Verification items for the finished model (mm, model axes). Face numbers are marked on the shaded views. A direction names the side the tool comes from. Give positions to 0.01 mm unless a question says otherwise; leave off trailing zeros. Order: outer loops, then holes, each group sorted by start corner. A loop starts at its lowest first (then second) coordinate and runs counter-clockwise, first axis right, second up.
(1) Sectioned sample at B-B on z = -0.75. Record the cut outline in (x, y).
(2) Access from +Z, -Z, +X, -X, +Y, -Y to the whole of each face (thin tool, end or side, straight path). Record for the marked faces 5, 6 and 7.
(3) Gauge pin test, flat ends, axial feed: pin 1 (3.5 mm diameter, centred on x = 5, y = -11.5, fed in from -Z); pin 2 (1.3 mm diameter, centred on y = 12, z = -3, fed in from -X); pin 3 (3.5 mm diameter, centred on y = 1.5, z = -0.5, fed in from -X); pin 4 (2 mm diameter, centred on x = 2, z = -3.5, fed in from -Y). Record the tip position at first contact, or that the pin passes through.
(4) Sectioned sample at A-A on x = -9.75. Record the cut outline in (y, z).
(5) Sectioned sample at D-D on x = 7. Record the cut outline in (y, z), plus the area to 3 significant figures.
(6) Mould release check, pull along Y, two halves, no side actions. Record for the marked faces 1, 2, 3 and 4: pulls with the +Y half, pulls with the -Y half, needs draft (parallel to the pull), parting line crosses it, or undercut.
(7) Sectioned sample at C-C on x = 3. Record the cut outline in (y, z), plus the area to 3 significant figures.
(8) Scan lines: L1, parallel to Y at x = 12.5, z = 0; L2, parallel to Y at x = -9.75, z = -4.25; L3, parallel to X at y = -1.25, z = 1.25. Record each from-to range of solid material in increasing order.
```python
from build123d import *

# Parameters (mm, degrees)
SKETCH1_W           = 30
SKETCH1_H           = 22
BOSS_EXTRUDE1_DEPTH = 2
SKETCH2_W           = 13
SKETCH2_H           = 20
CUT_EXTRUDE1_DEPTH  = 2
FILLET1_R           = 3
SKETCH3_W           = 30
SKETCH3_H           = 22
BOSS_EXTRUDE2_DEPTH = 20
SKETCH4_W           = 30
SKETCH4_H           = 22
BOSS_EXTRUDE3_DEPTH = 2
SKETCH5_W           = 30
SKETCH5_H           = 22
BOSS_EXTRUDE4_DEPTH = 2
SKETCH6_W           = 18.015144258
SKETCH6_H           = 26
CUT_EXTRUDE2_DEPTH  = 1.2
SKETCH7_W           = 18
SKETCH7_H           = 26
CUT_EXTRUDE3_DEPTH  = 1.2
SKETCH8_W           = 27.6
SKETCH8_H           = 18
CUT_EXTRUDE4_DEPTH  = 1.2
SKETCH9_W           = 27.6
SKETCH9_H           = 18.015144258
CUT_EXTRUDE5_DEPTH  = 1.2
SKETCH10_W          = 8.9
SKETCH10_H          = 1
CUT_EXTRUDE7_DEPTH  = 1.8
SKETCH12_W          = 5.2
SKETCH12_H          = 1.2
CUT_EXTRUDE8_DEPTH  = 1.8
CUT_EXTRUDE9_DEPTH  = 3.2
SKETCH14_W          = 2.8
SKETCH14_H          = 1
CUT_EXTRUDE10_DEPTH = 5
SKETCH15_W          = 8.9
SKETCH15_H          = 1
CUT_EXTRUDE11_DEPTH = 5
SKETCH16_W          = 5.1
SKETCH16_H          = 1.2
CUT_EXTRUDE12_DEPTH = 5
SKETCH17_W          = 27.6
SKETCH17_H          = 14.5
CUT_EXTRUDE13_DEPTH = 23.6
CUT_EXTRUDE14_DEPTH = 5
SKETCH19_W          = 2.8
SKETCH19_H          = 20
CUT_EXTRUDE16_DEPTH = 3.5
SKETCH20_W          = 8.574892863
SKETCH20_H          = 20
SKETCH20_W_2        = 12.614156469
CUT_EXTRUDE18_DEPTH = 5
SKETCH24_W          = 0.5
SKETCH24_H          = 26
CUT_EXTRUDE19_DEPTH = 100
SKETCH25_W          = 4.142834468
SKETCH25_H          = 28.533772401
SKETCH25_W_2        = 4.453547053
SKETCH25_H_2        = 29.155197571
CUT_EXTRUDE20_DEPTH = 3.5


with BuildPart() as part:
    # Sketch1 → Boss-Extrude1 (new body)
    with BuildSketch(Plane.XY):
        with Locations((1.554069904, 0.785714286)):
            Rectangle(SKETCH1_W, SKETCH1_H)
    extrude(amount=BOSS_EXTRUDE1_DEPTH)

    # Sketch2 → Cut-Extrude1 (cut)
    with BuildSketch(Plane.XY.offset(2)):
        with Locations((-5.945930096, 0.785714286)):
            Rectangle(SKETCH2_W, SKETCH2_H)
        with Locations((9.054069904, 0.785714286)):
            Rectangle(SKETCH2_W, SKETCH2_H)
    extrude(amount=-CUT_EXTRUDE1_DEPTH, mode=Mode.SUBTRACT)

    # Fillet1
    fillet1_edges = [part.edges().sort_by_distance(p)[0] for p in [
        (-12.445930096, -9.214285714, 1),
        (-12.445930096, 10.785714286, 1),
        (0.554069904, 10.785714286, 1),
        (0.554069904, -9.214285714, 1),
        (15.554069904, 10.785714286, 1),
        (15.554069904, -9.214285714, 1),
        (2.554069904, -9.214285714, 1),
        (2.554069904, 10.785714286, 1),
    ]]
    fillet(fillet1_edges, radius=FILLET1_R)

    # Sketch3 → Boss-Extrude2 (add)
    with BuildSketch(Plane(origin=(0, 0, 0), x_dir=(-1, 0, 0), z_dir=(0, 0, -1))):
        with Locations((-1.554069904, 0.785714286)):
            Rectangle(SKETCH3_W, SKETCH3_H)
    extrude(amount=BOSS_EXTRUDE2_DEPTH)

    # Sketch4 → Boss-Extrude3 (add)
    with BuildSketch(Plane(origin=(0, 11.785714286, 0), x_dir=(1, 0, 0), z_dir=(0, 1, 0))):
        with Locations((1.554069904, 9)):
            Rectangle(SKETCH4_W, SKETCH4_H)
    extrude(amount=BOSS_EXTRUDE3_DEPTH)

    # Sketch5 → Boss-Extrude4 (add)
    with BuildSketch(Plane(origin=(0, -10.214285714, 0), x_dir=(-1, 0, 0), z_dir=(0, -1, 0))):
        with Locations((-1.554069904, 9)):
            Rectangle(SKETCH5_W, SKETCH5_H)
    extrude(amount=BOSS_EXTRUDE4_DEPTH)

    # Sketch6 → Cut-Extrude2 (cut)
    with BuildSketch(Plane(origin=(16.554069904, 0, 0), x_dir=(0, 0, -1), z_dir=(1, 0, 0))):
        with Locations((10.992427871, 0.785714286)):
            Rectangle(SKETCH6_W, SKETCH6_H)
    extrude(amount=-CUT_EXTRUDE2_DEPTH, mode=Mode.SUBTRACT)

    # Sketch7 → Cut-Extrude3 (cut)
    with BuildSketch(Plane.ZY.offset(13.445930096)):
        with Locations((-11, 0.785714286)):
            Rectangle(SKETCH7_W, SKETCH7_H)
    extrude(amount=-CUT_EXTRUDE3_DEPTH, mode=Mode.SUBTRACT)

    # Sketch8 → Cut-Extrude4 (cut)
    with BuildSketch(Plane(origin=(0, 13.785714286, 0), x_dir=(1, 0, 0), z_dir=(0, 1, 0))):
        with Locations((1.554069904, 11)):
            Rectangle(SKETCH8_W, SKETCH8_H)
    extrude(amount=-CUT_EXTRUDE4_DEPTH, mode=Mode.SUBTRACT)

    # Sketch9 → Cut-Extrude5 (cut)
    with BuildSketch(Plane.XZ.offset(12.214285714)):
        with Locations((1.554069904, -10.992427871)):
            Rectangle(SKETCH9_W, SKETCH9_H)
    extrude(amount=-CUT_EXTRUDE5_DEPTH, mode=Mode.SUBTRACT)

    # Sketch10 → Cut-Extrude7 (cut)
    with BuildSketch(Plane(origin=(0, 12.585714286, 0), x_dir=(1, 0, 0), z_dir=(0, 1, 0))):
        with Locations((-7.795930096, 2.5)):
            Rectangle(SKETCH10_W, SKETCH10_H)
        with Locations((10.904069904, 2.5)):
            Rectangle(SKETCH10_W, SKETCH10_H)
    extrude(amount=-CUT_EXTRUDE7_DEPTH, mode=Mode.SUBTRACT)

    # Sketch12 → Cut-Extrude8 (cut)
    with BuildSketch(Plane(origin=(0, 12.585714286, 0), x_dir=(1, 0, 0), z_dir=(0, 1, 0))):
        with Locations((-5.945930096, 2.6)):
            Rectangle(SKETCH12_W, SKETCH12_H)
        with Locations((9.054069904, 2.6)):
            Rectangle(SKETCH12_W, SKETCH12_H)
    extrude(amount=-CUT_EXTRUDE8_DEPTH, mode=Mode.SUBTRACT)

    # Sketch13 → Cut-Extrude9 (cut)
    with BuildSketch(Plane.XY):
        with BuildLine():
            Line((-9.445930096, 10.785714286), (-2.445930096, 10.785714286))
            ThreePointArc((-2.445930096, 10.785714286), (-0.324609753, 9.907034629), (0.554069904, 7.785714286))
            Line((0.554069904, 7.785714286), (0.554069904, -6.214285714))
            ThreePointArc((0.554069904, -6.214285714), (-0.324609753, -8.335606058), (-2.445930096, -9.214285714))
            Line((-2.445930096, -9.214285714), (-9.445930096, -9.214285714))
            ThreePointArc((-9.445930096, -9.214285714), (-11.56725044, -8.335606058), (-12.445930096, -6.214285714))
            Line((-12.445930096, -6.214285714), (-12.445930096, 7.785714286))
            ThreePointArc((-12.445930096, 7.785714286), (-11.56725044, 9.907034629), (-9.445930096, 10.785714286))
        make_face()
        with BuildLine():
            Line((5.554069904, 10.785714286), (12.554069904, 10.785714286))
            ThreePointArc((12.554069904, 10.785714286), (14.675390247, 9.907034629), (15.554069904, 7.785714286))
            Line((15.554069904, 7.785714286), (15.554069904, -6.214285714))
            ThreePointArc((15.554069904, -6.214285714), (14.675390247, -8.335606058), (12.554069904, -9.214285714))
            Line((12.554069904, -9.214285714), (5.554069904, -9.214285714))
            ThreePointArc((5.554069904, -9.214285714), (3.43274956, -8.335606058), (2.554069904, -6.214285714))
            Line((2.554069904, -6.214285714), (2.554069904, 7.785714286))
            ThreePointArc((2.554069904, 7.785714286), (3.43274956, 9.907034629), (5.554069904, 10.785714286))
        make_face()
    extrude(amount=-CUT_EXTRUDE9_DEPTH, mode=Mode.SUBTRACT)

    # Sketch14 → Cut-Extrude10 (cut)
    with BuildSketch(Plane(origin=(0, 10.785714286, 0), x_dir=(1, 0, 0), z_dir=(0, 1, 0))):
        with Locations((13.954069904, 2.5)):
            Rectangle(SKETCH14_W, SKETCH14_H)
        with Locations((-10.845930096, 2.5)):
            Rectangle(SKETCH14_W, SKETCH14_H)
    extrude(amount=-CUT_EXTRUDE10_DEPTH, mode=Mode.SUBTRACT)

    # Sketch15 → Cut-Extrude11 (cut)
    with BuildSketch(Plane(origin=(0, -11.014285714, 0), x_dir=(-1, 0, 0), z_dir=(0, -1, 0))):
        with Locations((7.795930096, 2.484855742)):
            Rectangle(SKETCH15_W, SKETCH15_H)
        with Locations((-10.904069904, 2.484855742)):
            Rectangle(SKETCH15_W, SKETCH15_H)
    extrude(amount=-CUT_EXTRUDE11_DEPTH, mode=Mode.SUBTRACT)

    # Sketch16 → Cut-Extrude12 (cut)
    with BuildSketch(Plane(origin=(0, -11.014285714, 0), x_dir=(-1, 0, 0), z_dir=(0, -1, 0))):
        with Locations((5.895930096, 2.584855742)):
            Rectangle(SKETCH16_W, SKETCH16_H)
        with Locations((-9.004069904, 2.584855742)):
            Rectangle(SKETCH16_W, SKETCH16_H)
    extrude(amount=-CUT_EXTRUDE12_DEPTH, mode=Mode.SUBTRACT)

    # Sketch17 → Cut-Extrude13 (cut)
    with BuildSketch(Plane(origin=(0, 12.585714286, 0), x_dir=(1, 0, 0), z_dir=(0, 1, 0))):
        with Locations((1.554069904, 12.75)):
            Rectangle(SKETCH17_W, SKETCH17_H)
    extrude(amount=-CUT_EXTRUDE13_DEPTH, mode=Mode.SUBTRACT)

    # Sketch18 → Cut-Extrude14 (cut)
    with BuildSketch(Plane.XY.offset(-3.2)):
        with BuildLine():
            Line((-12.445930096, 7.785714286), (-12.445930096, -6.214285714))
            ThreePointArc((-12.445930096, -6.214285714), (-11.56725044, -8.335606058), (-9.445930096, -9.214285714))
            Line((-9.445930096, -9.214285714), (-2.445930096, -9.214285714))
            ThreePointArc((-2.445930096, -9.214285714), (-0.324609753, -8.335606058), (0.554069904, -6.214285714))
            Line((0.554069904, -6.214285714), (0.554069904, 7.785714286))
            ThreePointArc((0.554069904, 7.785714286), (-0.324609753, 9.907034629), (-2.445930096, 10.785714286))
            Line((-2.445930096, 10.785714286), (-9.445930096, 10.785714286))
            ThreePointArc((-9.445930096, 10.785714286), (-11.56725044, 9.907034629), (-12.445930096, 7.785714286))
        make_face()
        with BuildLine():
            Line((5.554069904, 10.785714286), (12.554069904, 10.785714286))
            ThreePointArc((12.554069904, 10.785714286), (14.675390247, 9.907034629), (15.554069904, 7.785714286))
            Line((15.554069904, 7.785714286), (15.554069904, -6.214285714))
            ThreePointArc((15.554069904, -6.214285714), (14.675390247, -8.335606058), (12.554069904, -9.214285714))
            Line((12.554069904, -9.214285714), (5.554069904, -9.214285714))
            ThreePointArc((5.554069904, -9.214285714), (3.43274956, -8.335606058), (2.554069904, -6.214285714))
            Line((2.554069904, -6.214285714), (2.554069904, 7.785714286))
            ThreePointArc((2.554069904, 7.785714286), (3.43274956, 9.907034629), (5.554069904, 10.785714286))
        make_face()
    extrude(amount=-CUT_EXTRUDE14_DEPTH, mode=Mode.SUBTRACT)

    # Sketch19 → Cut-Extrude16 (cut)
    with BuildSketch(Plane(origin=(0, 0, -5.5), x_dir=(-1, 0, 0), z_dir=(0, 0, -1))):
        with Locations((-13.954069904, 0.785714286)):
            Rectangle(SKETCH19_W, SKETCH19_H)
        with Locations((10.845930096, 0.785714286)):
            Rectangle(SKETCH19_W, SKETCH19_H)
    extrude(amount=-CUT_EXTRUDE16_DEPTH, mode=Mode.SUBTRACT)

    # Sketch20 → Cut-Extrude18 (cut)
    with BuildSketch(Plane.XY.offset(2)):
        with Locations((-13.733376528, 0.785714286)):
            Rectangle(SKETCH20_W, SKETCH20_H)
        with Locations((18.861148139, 0.785714286)):
            Rectangle(SKETCH20_W_2, SKETCH20_H)
    extrude(amount=-CUT_EXTRUDE18_DEPTH, mode=Mode.SUBTRACT)

    # Sketch24 → Cut-Extrude19 (cut)
    with BuildSketch(Plane.ZY.offset(13.445930096)):
        with Locations((1.75, 0.785714286)):
            Rectangle(SKETCH24_W, SKETCH24_H)
    extrude(amount=-CUT_EXTRUDE19_DEPTH, mode=Mode.SUBTRACT)

    # Sketch25 → Cut-Extrude20 (cut)
    with BuildSketch(Plane.XY.offset(1.5)):
        with Locations((-14.51734733, 1.251783163)):
            Rectangle(SKETCH25_W, SKETCH25_H)
        with Locations((17.78084343, 0.941070578)):
            Rectangle(SKETCH25_W_2, SKETCH25_H_2)
    extrude(amount=-CUT_EXTRUDE20_DEPTH, mode=Mode.SUBTRACT)


solid = part.part
```
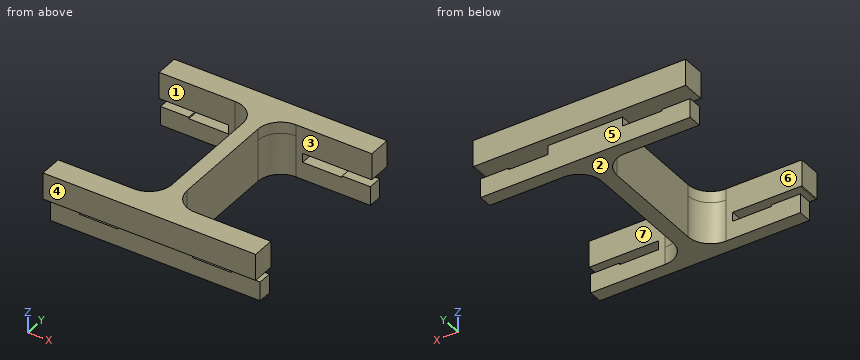
Ans:
1. outline: (-12.45, -12.21) - (15.55, -12.21) - (15.55, -9.21) - (5.55, -9.21) arc R3 cw to (2.55, -6.21) - (2.55, 7.79) arc R3 cw to (5.55, 10.79) - (15.55, 10.79) - (15.55, 13.79) - (-12.45, 13.79) - (-12.45, 10.79) - (-2.45, 10.79) arc R3 cw to (0.55, 7.79) - (0.55, -6.21) arc R3 cw to (-2.45, -9.21) - (-12.45, -9.21) - close
2. face 5: -Z, +X, -X, +Y
2. face 6: +Z, -Z, -X
2. face 7: +Z, -Z, +X
3. pin 1: stops at z = -5.5
3. pin 2: stops at x = -12.25
3. pin 3: stops at x = 0.55
3. pin 4: stops at y = -11.01
4. outline: (-12.21, -1.98) - (-9.21, -1.98) - (-9.21, 1.5) - (-12.21, 1.5) - close; (-11.01, -5.5) - (-9.21, -5.5) - (-9.21, -2.98) - (-11.01, -2.98) - close; (10.79, -5.5) - (12.59, -5.5) - (12.59, -3) - (10.79, -3) - close; (10.79, -2) - (13.79, -2) - (13.79, 1.5) - (10.79, 1.5) - close
5. outline: (-12.21, -1.98) - (-9.21, -1.98) - (-9.21, 1.5) - (-12.21, 1.5) - close; (-11.01, -5.5) - (-9.21, -5.5) - (-9.21, -3.18) - (-11.01, -3.18) - close; (10.79, -5.5) - (12.59, -5.5) - (12.59, -3.2) - (10.79, -3.2) - close; (10.79, -2) - (13.79, -2) - (13.79, 1.5) - (10.79, 1.5) - close
5. area: 29.3 mm2
6. face 1: undercut
6. face 2: needs draft
6. face 3: undercut
6. face 4: pulls with the -Y half
7. outline: (-12.21, -1.98) - (-11.01, -1.98) - (-11.01, -5.5) - (-7.79, -5.5) - (-7.79, 1.5) - (-12.21, 1.5) - close; (9.36, -5.5) - (12.59, -5.5) - (12.59, -2) - (13.79, -2) - (13.79, 1.5) - (9.36, 1.5) - close
7. area: 53.5 mm2
8. L1: y = -12.21 to -9.21, 10.79 to 13.79
8. L2: y = -11.01 to -9.21, 10.79 to 12.59
8. L3: x = 0.55 to 2.55
